Autodesk Inventor part; units mm, degrees
ref_plane "YZ Plane" through (0, 0, 0) normal (1, 0, 0) x (0, 1, 0)
ref_plane "XZ Plane" through (0, 0, 0) normal (0, 1, 0) x (-1, 0, 0)
ref_plane "XY Plane" through (0, 0, 0) normal (0, 0, 1) x (1, 0, 0)
sketch "Sketch1" plane through (0, 0, 0) normal (0, 1, 0) x (-1, 0, 0)
  line L0 (-3.175, -3.175) -> (3.175, -3.175)
  line L1 (3.175, -3.175) -> (3.175, 3.175)
  line L2 (3.175, 3.175) -> (-3.175, 3.175)
  line L3 (-3.175, 3.175) -> (-3.175, -3.175)
  line L4 (-3.175, -3.175) -> (3.175, 3.175) construction
  line L5 (3.175, -3.175) -> (-3.175, 3.175) construction
  point P0 (0, 0)
  dimension "d0" = 6.35
  dimension "d1" = 6.35
extrude "Extrusion1" add sketch "Sketch1" along normal blind 76.2
sketch "Sketch2" plane through (3.175, 0, 3.175) normal (1, 0, 0) x (0, 0, -1)
  circle A0 centre (3.175, 3.175) radius 2.159
  line L0 (0, 0) -> (6.35, 0)
  point P0 (3.175, 0)
  dimension "d4" = 4.318
  dimension "d5" = 3.175
extrude "Extrusion2" cut sketch "Sketch2" against normal blind 76.2
fillet "Fillet1" radius 1.5875 4 edges at (3.175, 38.1, -3.175) (-3.175, 38.1, -3.175) (3.175, 38.1, 3.175) (-3.175, 38.1, 3.175)
fillet "Fillet2" radius 0.7937 16 edges at (2.71, 0, 2.71) (3.175, 0, 0) (2.71, 0, -2.71) (0, 0, -3.175) (-2.71, 0, -2.71) (-3.175, 0, 0) (-2.71, 0, 2.71) (0, 0, 3.175) (2.71, 76.2, 2.71) (3.175, 76.2, 0) (2.71, 76.2, -2.71) (0, 76.2, -3.175) (-2.71, 76.2, -2.71) (-3.175, 76.2, 0) (-2.71, 76.2, 2.71) (0, 76.2, 3.175)
sketch "Sketch3" plane through (-1.5875, 75.4062, 3.175) normal (0, 0, 1) x (1, 0, 0)
  circle A0 centre (1.5875, -44.9263) radius 2.159
  line L0 (0, -75.4062) -> (3.175, -75.4062)
  point P0 (1.5875, -75.4062)
  dimension "d10" = 4.318
  dimension "d11" = 30.48
extrude "Extrusion3" cut sketch "Sketch3" against normal blind 76.2
sketch "Sketch4" plane through (-1.5875, 75.4062, 3.175) normal (0, 0, 1) x (1, 0, 0)
  circle A0 centre (1.5875, -2.3813) radius 2.159
  line L0 (3.175, 0.7937) -> (0, 0.7937)
  point P0 (1.5875, -75.4062)
  dimension "d14" = 4.318
  dimension "d15" = 3.175
extrude "Extrusion4" cut sketch "Sketch4" against normal blind 76.2
properties part number "beam" material "Stainless Steel"
Here's how the part is built. I have some questions about the finished solid (model axes, mm). A direction names the side the tool comes from. Give positions to 0.01 mm unless a question says otherwise; leave off trailing zeros. Write each loop counter-clockwise with the first axis right and the second up, starting at its lowest first coordinate (ties: lowest second). Pieces come first, ordered by that corner, then holes. Notation, with made-up numbers: (-24, -12) -> (32, -12) arc R6 cw to (32, -7) -> close; hole circle Ø10 at (56, 5). An arc over 180 degrees is marked (long way). Write each question's results on one line, items separated by ' | '.
Item 1: Suppose I cut it at A-A on x = 0. Write out the boundary of the cut face in (y, z) (3 decimals).
Output:
outline: (0, -2.381) arc R0.794 ccw to (0.794, -3.175) -> (28.321, -3.175) -> (28.321, 3.175) -> (0.794, 3.175) arc R0.794 ccw to (0, 2.381) -> close; (32.639, -3.175) -> (70.866, -3.175) -> (70.866, 3.175) -> (32.639, 3.175) -> close; (75.184, -3.175) -> (75.406, -3.175) arc R0.794 ccw to (76.2, -2.381) -> (76.2, 2.381) arc R0.794 ccw to (75.406, 3.175) -> (75.184, 3.175) -> close; hole circle Ø4.318 at (3.175, 0)
Item 2: We'd pull the mould along Y, two halves only. Please class faces 4 (the face through (0, 0, 0)), 5 (the face through (2.7, 1.26, 2.72)), 6 (the face through (0, 76.2, 0)), 7 (the face through (0.044, 1.067, 0.468)): pulls with the +Y half, pulls with the -Y half, needs draft (parallel to the pull), parting line crosses it, or undercut.
Output:
face 4: pulls with the -Y half | face 5: needs draft | face 6: pulls with the +Y half | face 7: undercut
Item 3: Suppose I cut it at B-B on z = 0.25. Write out the boundary of the cut face in (x, y) (3 decimals).
Output:
outline: (-3.175, 0.794) arc R0.794 ccw to (-2.381, 0) -> (2.381, 0) arc R0.794 ccw to (3.175, 0.794) -> (3.175, 1.031) -> (-3.175, 1.031) -> close; (-3.175, 5.319) -> (3.175, 5.319) -> (3.175, 75.406) arc R0.794 ccw to (2.381, 76.2) -> (-2.381, 76.2) arc R0.794 ccw to (-3.175, 75.406) -> close; hole circle Ø4.318 at (0, 30.48); hole circle Ø4.318 at (0, 73.025)
Item 4: On a 3-axis mill with a long thin cutter (end or side, diameter ignored), from which of +Z, -Z, +X, -X, +Y, -Y can I reach the whole of each face in a straight line? I mean faces 1 (the face through (2.7, 40.52, 2.72)), 2 (the face through (-2.72, 40.52, 2.7)), 3 (the face through (2.72, 1.26, -2.7)). Say none if no direction works.
Output:
face 1: +Z, +X, +Y | face 2: +Z, -X, +Y | face 3: -Z, +X, -Y
Item 5: Suppose I cut it at C-C on y = 39. Write out the boundary of the cut face in (x, z) (1 decimal).
Output:
outline: (-3.2, -1.6) arc R1.6 ccw to (-1.6, -3.2) -> (1.6, -3.2) arc R1.6 ccw to (3.2, -1.6) -> (3.2, 1.6) arc R1.6 ccw to (1.6, 3.2) -> (-1.6, 3.2) arc R1.6 ccw to (-3.2, 1.6) -> close
Item 6: If I drill on L1, parallel to Z at x = -1.25, y = 4.5 (3 decimals); L2, parallel to Y at x = 0.25, z = 0; L3, parallel to Y at x = -0.5, z = 3, over which ranges is the centre line in solid material (lowest first)?
Output:
L1: z = -3.175 to -1.705, 1.705 to 3.175 | L2: y = 0 to 1.02, 5.33 to 28.34, 32.62 to 70.88, 75.17 to 76.2 | L3: y = 0.3 to 28.38, 32.58 to 70.92, 75.13 to 75.9
